Read the model definition and answer for the solid it produces. Units are mm, in the model's axes. Face numbers are marked on the shaded views. A direction names the side the tool comes from. Coordinates: 2 decimals unless noted, no trailing zeros. Order: outer loops, then holes, each group sorted by start corner. A loop starts at its lowest first (then second) coordinate and runs counter-clockwise, first axis right, second up. Notation, with made-up numbers: M 28.25,46.5 L 67.25,46.5 A31 cw 67.25,76.5 Z; hole C -24,-21 d11. An arc over 180 degrees is marked long. Put each result on its own line as item: value.
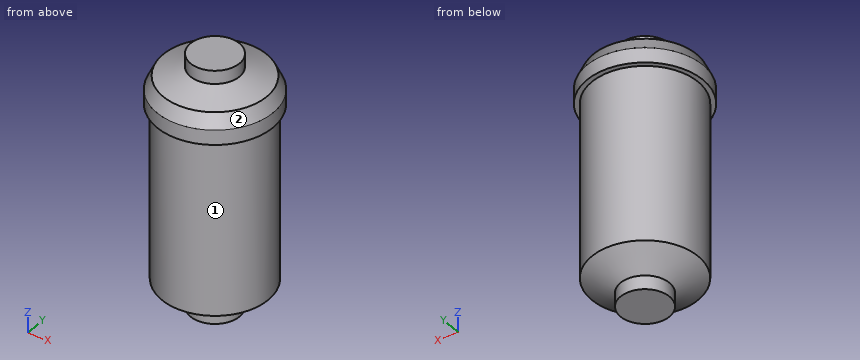
from build123d import *

# Parameters (mm, degrees)
SKETCH1_R           = 14.732
BOSS_EXTRUDE1_DEPTH = 8.255
SKETCH2_R           = 14.732
SKETCH3_R           = 32.004
SKETCH4_R           = 32.004
BOSS_EXTRUDE2_DEPTH = 104.9655
SKETCH5_R           = 34.925
BOSS_EXTRUDE3_DEPTH = 8.89
SKETCH6_R           = 34.925
SKETCH7_R           = 31.115
SKETCH8_R           = 31.115
SKETCH9_R           = 14.732
SKETCH10_R          = 14.732
BOSS_EXTRUDE4_DEPTH = 7.9375


with BuildPart() as part:
    # Sketch1 → Boss-Extrude1 (new body)
    with BuildSketch(Plane.XY):
        Circle(SKETCH1_R)
    extrude(amount=BOSS_EXTRUDE1_DEPTH)

    # Sketch2 → Loft1 section 0
    with BuildSketch(Plane.XY.offset(8.255)):
        Circle(SKETCH2_R)
    # Sketch3 → Loft1 section 1
    with BuildSketch(Plane.XY.offset(17.145)):
        Circle(SKETCH3_R)
    loft()

    # Sketch4 → Boss-Extrude2 (add)
    with BuildSketch(Plane.XY.offset(17.145)):
        Circle(SKETCH4_R)
    extrude(amount=BOSS_EXTRUDE2_DEPTH)

    # Sketch5 → Boss-Extrude3 (add)
    with BuildSketch(Plane.XY.offset(122.1105)):
        Circle(SKETCH5_R)
    extrude(amount=BOSS_EXTRUDE3_DEPTH)

    # Sketch6 → Loft2 section 0
    with BuildSketch(Plane.XY.offset(131.0005)):
        Circle(SKETCH6_R)
    # Sketch7 → Loft2 section 1
    with BuildSketch(Plane.XY.offset(139.1285)):
        Circle(SKETCH7_R)
    loft()

    # Sketch8 → Loft3 section 0
    with BuildSketch(Plane.XY.offset(139.1285)):
        Circle(SKETCH8_R)
    # Sketch9 → Loft3 section 1
    with BuildSketch(Plane.XY.offset(144.4625)):
        Circle(SKETCH9_R)
    loft()

    # Sketch10 → Boss-Extrude4 (add)
    with BuildSketch(Plane.XY.offset(144.4625)):
        Circle(SKETCH10_R)
    extrude(amount=BOSS_EXTRUDE4_DEPTH)


solid = part.part
Q1. Consider line 1 along Y through (x, z) = (6, 146); line 2 along Z through (x, y) = (25.5, 23.5); line 3 along X through (y, z) = (13, 146). Determine where each line is inside the solid, lowest interval first.
Answers below:
line 1: y = -13.45 to 13.45
line 2: z = 122.11 to 131.53
line 3: x = -6.93 to 6.93
Q2. Find section A-A on x = 0. Write down the section's boundary in (y, z) (1 decimal), plus the area to 3 significant figures.
Answers below:
outline: M -34.9,122.1 L -32,122.1 L -32,17.1 L -14.7,8.3 L -14.7,0 L 14.7,0 L 14.7,8.3 L 32,17.1 L 32,122.1 L 34.9,122.1 L 34.9,131 L 31.1,139.1 L 14.7,144.5 L 14.7,152.4 L -14.7,152.4 L -14.7,144.5 L -31.1,139.1 L -34.9,131 Z
area: 9,010 mm^2
Q3. Given pin 1 (3 mm diameter, centred on x = 26.5, z = 105.5, fed in from -Y); pin 2 (1.5 mm diameter, centred on x = -14.5, z = 27, fed in from +Y); pin 3 (21 mm diameter, centred on x = -16, y = -17.5, fed in from -Z); pin 4 (4 mm diameter, centred on x = -20, y = 16.5, fed in from +Z), each flat-ended and moving along its own axis, determine where each tip first touches the part or whether it passes through.
Answers below:
pin 1: stops at y = -19.98
pin 2: stops at y = 28.9
pin 3: stops at z = 0
pin 4: stops at z = 141.47
Q4. A tool of negligible diameter and unlimited length cuts with its end or side. For the marked faces 1 and 2, from which of +Z, -Z, +X, -X, +Y, -Y can it reach the whole face along a straight path? Write none if from no direction.
Answers below:
face 1: -Z
face 2: +Z
Q5. Find section B-B on z = 57.5. Write down the section's boundary in (x, y).
Answers below:
outline: C 0,0 d64.01
